Geometry check sheet. Reference: the model listing, model coordinates, mm. A direction names the side the tool comes from. Give positions to 0.01 mm unless a question says otherwise; leave off trailing zeros. Order: outer loops, then holes, each group sorted by start corner. A loop starts at its lowest first (then second) coordinate and runs counter-clockwise, first axis right, second up. Notation, with made-up numbers: (-32, 48.5) - (26, 48.5) arc R20 cw to (26, 87.5) - close; hole circle Ø8 at (58, 77). An arc over 180 degrees is marked (long way). Put each result on its own line as item: value. Start each with the question number.
```python
from build123d import *

# Parameters (mm, degrees)
F1_DEPTH = 1
F2_DEPTH = 11
F3_R     = 5
F4_R     = 3
F5_R     = 3
F6_DEPTH = 2
F7_R     = 1


with BuildPart() as f1:
    # F0 (on Top) → F1 (new body)
    with BuildSketch(Plane.XY):
        Polygon((41, -16.9827560573), (41, 16.9827560573), (16.9827560573, 41), (-16.9827560573, 41), (-41, 16.9827560573), (-41, -16.9827560573), (-16.9827560573, -41), (-16.9827560573, -48), (16.9827560573, -48), (16.9827560573, -41), align=None)
        Polygon((-33, -13.6690475583), (-33, 13.6690475583), (-13.6690475583, 33), (13.6690475583, 33), (33, 13.6690475583), (33, -13.6690475583), (13.6690475583, -33), (-13.6690475583, -33), align=None, mode=Mode.SUBTRACT)
    extrude(amount=F1_DEPTH)

    # F0 (on Top) → F2 (join)
    with BuildSketch(Plane.XY):
        Polygon((-17.3969696197, 42), (-42, 17.3969696197), (-42, -17.3969696197), (-18.4827560573, -40.9142135624), (-18.4827560573, -49.5), (18.3969696197, -49.5), (18.3969696197, -41), (42, -17.3969696197), (42, 17.3969696197), (17.3969696197, 42), align=None)
        Polygon((16.9827560573, 41), (41, 16.9827560573), (41, -16.9827560573), (16.9827560573, -41), (16.9827560573, -48), (-16.9827560573, -48), (-16.9827560573, -41), (-41, -16.9827560573), (-41, 16.9827560573), (-16.9827560573, 41), align=None, mode=Mode.SUBTRACT)
        Polygon((-13.6690475583, 33), (-33, 13.6690475583), (-33, -13.6690475583), (-13.6690475583, -33), (13.6690475583, -33), (33, -13.6690475583), (33, 13.6690475583), (13.6690475583, 33), align=None)
        Polygon((-32, 13.2548339959), (-13.2548339959, 32), (13.2548339959, 32), (32, 13.2548339959), (32, -13.2548339959), (13.2548339959, -32), (-13.2548339959, -32), (-32, -13.2548339959), align=None, mode=Mode.SUBTRACT)
    extrude(amount=F2_DEPTH)

    # F3
    f3_edges = [f1.edges().sort_by_distance(p)[0] for p in [
        (-42, 17.39697, 5.5),
        (-42, -17.39697, 5.5),
        (-17.39697, 42, 5.5),
        (17.39697, 42, 5.5),
        (42, 17.39697, 5.5),
        (42, -17.39697, 5.5),
        (-13.254834, 32, 5.5),
        (-32, 13.254834, 5.5),
        (-32, -13.254834, 5.5),
        (-13.254834, -32, 5.5),
        (13.254834, -32, 5.5),
        (32, -13.254834, 5.5),
        (32, 13.254834, 5.5),
        (13.254834, 32, 5.5),
        (18.39697, -41, 5.5),
        (-18.482756, -40.914214, 5.5),
    ]]
    fillet(f3_edges, radius=F3_R)

    # F4
    f4_edges = [f1.edges().sort_by_distance(p)[0] for p in [
        (-33, -13.669048, 6),
        (-13.669048, -33, 6),
        (13.669048, -33, 6),
        (33, -13.669048, 6),
        (33, 13.669048, 6),
        (13.669048, 33, 6),
        (-13.669048, 33, 6),
        (-33, 13.669048, 6),
        (41, -16.982756, 6),
        (41, 16.982756, 6),
        (16.982756, 41, 6),
        (-16.982756, 41, 6),
        (-41, 16.982756, 6),
        (-41, -16.982756, 6),
        (-16.982756, -41, 6),
        (16.982756, -41, 6),
        (18.39697, -49.5, 5.5),
        (-18.482756, -49.5, 5.5),
    ]]
    fillet(f4_edges, radius=F4_R)

    # F5 (on face) → F6 (cut)
    with BuildSketch(Plane.XZ.offset(49.5)):
        with Locations((0, 5.5)):
            Circle(F5_R)
    extrude(amount=-F6_DEPTH, mode=Mode.SUBTRACT)

    # F7
    f7_edges = [f1.edges().sort_by_distance(p)[0] for p in [
        (-16.982756, -48, 6),
        (16.982756, -48, 6),
    ]]
    fillet(f7_edges, radius=F7_R)


solid = f1.part
```
Item 1: Cross-section at D-D (x = -29). Enter the section's corners in (y, z).
Item 2: Gauge pin test, flat ends, axial feed: pin 1 Ø3 at (y, z) = (-44.5, 4) entering from -X; pin 2 Ø4 at (x, z) = (-29.5, 5.5) entering from +Y; pin 3 Ø5.5 at (x, z) = (0, 5.5) entering from -Y. Record the tip position at first contact, or that the pin passes through.
Item 3: Cross-section at C-C (z = 5.5). Count the separate pieces of the cut face and the enclosed holes in it, and give its area (3 significant figures).
Item 4: Thickness scan on line 1 along Y through (x, z) = (11, 4.5); line 2 along X through (y, z) = (29, 10.5); line 3 along X through (y, z) = (-18, 4). Record the ranges inside material, lowest first.
Item 5: Release check for a two-part mould opening along Z. For faces 4 (the face through (-18.874, -41.046, 5.577)), 5 (the face through (-0.65, -48.76, 2.57)), 6 (the face through (-24, -23, 1)) record: +Z half, -Z half, draft (parallel to the pull), parting line (faces both ways), or undercut.
Item 6: Cross-section at A-A (y = 7). Enter the section's corners in (x, z).
Item 7: Set-up check for faces 1 (the face through (41.63, -17.21, 5.58)), 2 (the face through (13.559, 32.778, 6.07)), 3 (the face through (22.738, -22.517, 5.423)): record each of +Z, -Z, +X, -X, +Y, -Y from which the full face is reachable in a straight line by a thin tool's end or side.
Item 8: Cross-section at B-B (x = 0). Enter the section's corners in (y, z), and give its area (3 significant figures).
Recorded:
1. outline: (-30.4, 0) - (-16.25, 0) - (-16.25, 11) - (-17.67, 11) - (-17.67, 1) - (-28.98, 1) - (-28.98, 11) - (-30.4, 11) - close; (16.25, 0) - (30.4, 0) - (30.4, 11) - (28.98, 11) - (28.98, 1) - (17.67, 1) - (17.67, 11) - (16.25, 11) - close
2. pin 1: stops at x = -18.48
2. pin 2: stops at y = 31.9
2. pin 3: stops at y = -33
3. separate pieces: 2
3. enclosed holes: 1
3. area: 519 mm^2
4. line 1: y = -49.5 to -48, -33 to -32, 32 to 33, 41 to 42
4. line 2: x = -30.4 to -28.98, -17.67 to -16.25, 16.25 to 17.67, 28.98 to 30.4
4. line 3: x = -41.22 to -39.98, -28.67 to -27.25, 27.25 to 28.67, 39.98 to 41.22
5. face 4: draft
5. face 5: undercut
5. face 6: +Z half
6. outline: (-42, 0) - (-32, 0) - (-32, 11) - (-33, 11) - (-33, 1) - (-41, 1) - (-41, 11) - (-42, 11) - close; (32, 0) - (42, 0) - (42, 11) - (41, 11) - (41, 1) - (33, 1) - (33, 11) - (32, 11) - close
7. face 1: +Z, -Z, +X, -Y
7. face 2: +Z
7. face 3: +Z, -Z
8. outline: (-49.5, 0) - (-32, 0) - (-32, 11) - (-33, 11) - (-33, 1) - (-48, 1) - (-48, 2.5) - (-49.5, 2.5) - close; (-49.5, 8.5) - (-48, 8.5) - (-48, 11) - (-49.5, 11) - close; (32, 0) - (42, 0) - (42, 11) - (41, 11) - (41, 1) - (33, 1) - (33, 11) - (32, 11) - close
8. area: 63.5 mm^2
